from build123d import *

# Parameters (mm, degrees)
EXTRUDE_1_DEPTH = 10
EXTRUDE_2_DEPTH = 20


with BuildPart() as part:
    # Sketch 1 → Extrude 1 (new body)
    with BuildSketch(Plane(origin=(0, 0, 0), x_dir=(1, 0, 0), z_dir=(0, 1, 0))):
        with BuildLine():
            Line((15, 10), (5, 10))
            Line((5, 10), (5, 5))
            Line((5, 5), (0, 5))
            ThreePointArc((0, 5), (-5, 0), (0, -5))
            Line((0, -5), (5, -5))
            Line((5, -5), (5, -10))
            Line((5, -10), (15, -10))
            Line((15, -10), (15, -5))
            ThreePointArc((15, -5), (10, 0), (15, 5))
            Line((15, 5), (15, 10))
        make_face()
        with BuildLine():
            Line((5, 5), (5, 10))
            Line((5, 10), (0, 10))
            ThreePointArc((0, 10), (-10, 0), (0, -10))
            Line((0, -10), (5, -10))
            Line((5, -10), (5, -5))
            Line((5, -5), (0, -5))
            ThreePointArc((0, -5), (-5, 0), (0, 5))
            Line((0, 5), (5, 5))
        make_face()
    extrude(amount=EXTRUDE_1_DEPTH)

    # Sketch 1_3 → Extrude 2 (add)
    with BuildSketch(Plane(origin=(0, 0, 0), x_dir=(1, 0, 0), z_dir=(0, 1, 0))):
        with BuildLine():
            Line((5, 5), (5, 10))
            Line((5, 10), (0, 10))
            ThreePointArc((0, 10), (-10, 0), (0, -10))
            Line((0, -10), (5, -10))
            Line((5, -10), (5, -5))
            Line((5, -5), (0, -5))
            ThreePointArc((0, -5), (-5, 0), (0, 5))
            Line((0, 5), (5, 5))
        make_face()
    extrude(amount=EXTRUDE_2_DEPTH)


solid = part.part
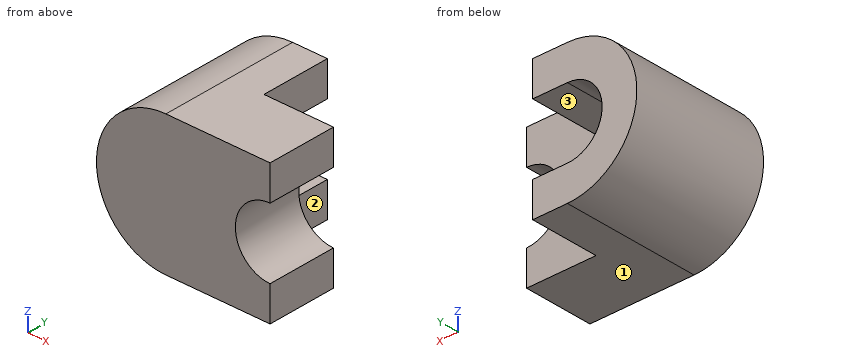
Build history of the part. All positions in model axes, mm. Face numbers are marked on the shaded views. A direction names the side the tool comes from. Round coordinates to 2 decimals unless told otherwise and drop trailing zeros. Write each loop counter-clockwise with the first axis right and the second up, starting at its lowest first coordinate (ties: lowest second). Pieces come first, ordered by that corner, then holes. Notation, with made-up numbers: M 61,88 L 79,88 A30 cw 79,111 Z; hole C 38,69 d7. An arc over 180 degrees is marked long. Answer in a Markdown table with one row per item.
1. Saw through at D-D (x = 5.75). List the corners of the cut face in (y, z), and give its area (3 significant figures).
Geometry check:
| item | result |
|---|---|
| outline | M 0,-10 L 10,-10 L 10,10 L 0,10 Z |
| area | 200 mm2 |
2. Saw through at C-C (y = 13.5). List the corners of the cut face in (x, z).
Geometry check:
| item | result |
|---|---|
| outline | M 0,-10 L 5,-10 L 5,-5 L 0,-5 A5 cw 0,5 L 5,5 L 5,10 L 0,10 A10 ccw Z |
3. Flat gauge pins, fed straight in: P1, Ø10, axis at y = 14.5, z = 1, coming from the +X side; P2, Ø5, axis at y = 17, z = -6, coming from the +X side; P3, Ø3, axis at y = 17.5, z = 1, coming from the +X side. Where does each tip first touch, or does it go through?
Geometry check:
| item | result |
|---|---|
| P1 | x = 11.14 |
| P2 | x = 5 |
| P3 | x = -4.33 |
4. Saw through at B-B (z = 0). List the corners of the cut face in (x, y).
Geometry check:
| item | result |
|---|---|
| outline | M -10,0 L 10,0 L 10,10 L -5,10 L -5,20 L -10,20 Z |
5. Saw through at A-A (x = 12.75). List the corners of the cut face in (y, z).
Geometry check:
| item | result |
|---|---|
| outline | M 0,-10 L 10,-10 L 10,-4.47 L 0,-4.47 Z; M 0,4.47 L 10,4.47 L 10,10 L 0,10 Z |
6. Probe L1, parallel to Z at x = 1, y = 14; L2, parallel to Y at x = 5.75, z = -8.75; L3, parallel to Z at x = -0.75, y = 15. List the from-to ranges inside material, lowest first. Write a range as [from, to].
Geometry check:
| item | result |
|---|---|
| L1 | [-10, -5], [5, 10] |
| L2 | [0, 10] |
| L3 | [-9.97, -4.94], [4.94, 9.97] |
7. Which spindle directions (+Z, -Z, +X, -X, +Y, -Y) get a long thin tool onto all of the face, cutting with end or side? Do the marked faces 1, 2 and 3. Say none if no direction does.
Geometry check:
| item | result |
|---|---|
| face 1 | -Z, +X, -X, +Y, -Y |
| face 2 | +Z, -Z, +X, +Y |
| face 3 | +X, +Y |
